Here's the drawing with two shaded views (mm, measured from the low corner). I have some questions. A direction names the side the tool comes from. Coordinates: 2 decimals unless noted, no trailing zeros. Write each loop counter-clockwise with the first axis right and the second up, starting at its lowest first coordinate (ties: lowest second). Pieces come first, ordered by that corner, then holes. Notation, with made-up numbers: M 0,83.5 L 56,83.5 A28 cw 56,117.5 Z; hole C 74,72 d5. An arc over 180 degrees is marked long. Use one line per item in the form item = value. Start each with the question number.
1. I'm going to push flat-ended pins straight in: pin 1 Ø0.8 at (y, z) = (1, 5.5) entering from -X; pin 2 Ø0.8 at (x, z) = (1, 9) entering from -Y; pin 3 Ø0.8 at (x, y) = (2.5, 3) entering from +Z. Where does each tip first touch, or does it pass through?
2. I want a section at D-D, the plane z = 4.25. List the corners of the cut face in (x, y) for me, plus the area to 3 significant figures.
3. I want a section at B-B, the plane z = 12. List the corners of the cut face in (x, y) for me, plus the area to 3 significant figures.
4. I want a section at A-A, the plane y = 0.95. List the corners of the cut face in (x, z) for me, plus the area to 3 significant figures.
5. Thinking about a two-plate mould opening in X: for the marked faces 6, 7 and 8, which applies, released by +X, released by -X, zero draft, split by the parting line, or undercut?
6. I want a section at C-C, the plane x = 10. List the corners of the cut face in (y, z) for me, plus the area to 3 significant figures.
7. Please list where these lines run through material, in increasing order: line 1 along X through (y, z) = (1.85, 5.75); line 2 along Y through (x, z) = (2.5, 13); line 3 along X through (y, z) = (1.05, 0.5). Write a range as [from, to].
8. On a 3-axis mill with a long thin cutter (end or side, diameter ignored), from which of +Z, -Z, +X, -X, +Y, -Y can I reach the whole of each face in a straight line? I mean the marked faces 1, 2, 3, 4 and 5. Say none if no direction works.
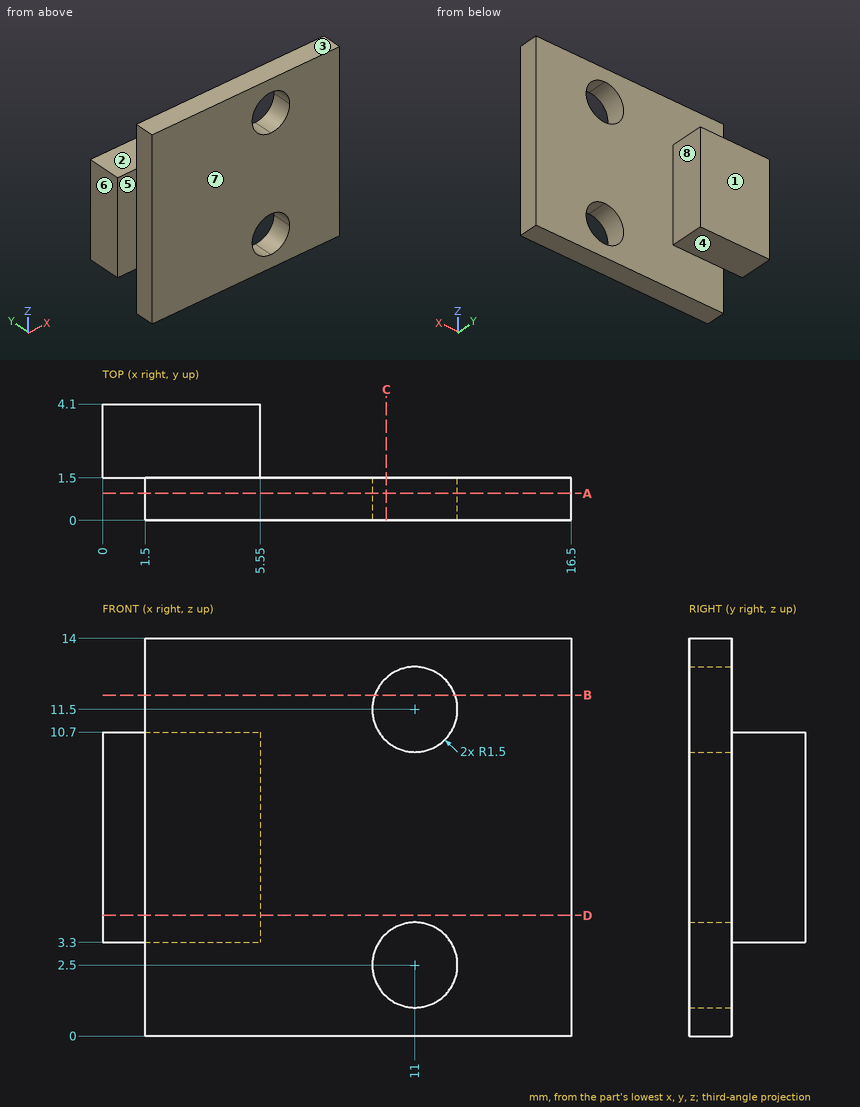
Answer list:
q1.pin_1 = 1.5
q1.pin_2 = 1.5
q1.pin_3 = 10.7
q2.outline = M 0,1.5 L 1.5,1.5 L 1.5,0 L 16.5,0 L 16.5,1.5 L 5.55,1.5 L 5.55,4.1 L 0,4.1 Z
q2.area = 36.9 mm²
q3.outline = M 1.5,0 L 9.59,0 L 9.59,1.5 L 1.5,1.5 Z; M 12.41,0 L 16.5,0 L 16.5,1.5 L 12.41,1.5 Z
q3.area = 18.3 mm²
q4.outline = M 1.5,0 L 16.5,0 L 16.5,14 L 1.5,14 Z; hole C 11,2.5 d3; hole C 11,11.5 d3
q4.area = 196 mm²
q5.face_6 = released by -X
q5.face_7 = zero draft
q5.face_8 = released by +X
q6.outline = M 0,0 L 1.5,0 L 1.5,1.38 L 0,1.38 Z; M 0,3.62 L 1.5,3.62 L 1.5,10.38 L 0,10.38 Z; M 0,12.62 L 1.5,12.62 L 1.5,14 L 0,14 Z
q6.area = 14.3 mm²
q7.line_1 = [0, 5.55]
q7.line_2 = [0, 1.5]
q7.line_3 = [1.5, 16.5]
q8.face_1 = +Z, -Z, +X, -X, +Y
q8.face_2 = +Z, +X, -X, +Y
q8.face_3 = +Z, +X, -X, +Y, -Y
q8.face_4 = -Z, +X, -X, +Y
q8.face_5 = +Z, -Z, -X, -Y
